Check sheet for the modelled part. Datum: model origin and axes. Units: mm. A direction names the side the tool comes from. Round coordinates to 2 decimals unless told otherwise and drop trailing zeros. Write each loop counter-clockwise with the first axis right and the second up, starting at its lowest first coordinate (ties: lowest second). Pieces come first, ordered by that corner, then holes. Notation, with made-up numbers: (9, 59.25) -> (38, 59.25) arc R26 cw to (38, 90.25) -> close; hole circle Ø10 at (-19, 36.25). An arc over 180 degrees is marked (long way). Write item = value, one per line.
from build123d import *

# Parameters (mm, degrees)
SKETCH1_W                    = 35
SKETCH1_H                    = 35
SKETCH1_R                    = 2.25
BASE_FLANGE1_DEPTH           = 3
EDGE_FLANGE1_DEPTH           = 35
SKETCH9_W                    = 36
SKETCH9_H                    = 35
BOSS_EXTRUDE1_DEPTH          = 3
EDGE_FLANGE2_STRIP_W         = 18
EDGE_FLANGE2_STRIP_H         = 3
EDGE_FLANGE2_STRIP_CUT_DEPTH = 75
EDGE_FLANGE2_DEPTH           = 75
EDGE_FLANGE3_STRIP_W         = 18
EDGE_FLANGE3_STRIP_H         = 3
EDGE_FLANGE3_STRIP_CUT_DEPTH = 75
EDGE_FLANGE3_DEPTH           = 75
SKETCH16_R                   = 5.25
SKETCH16_R_2                 = 1.75
CUT_EXTRUDE1_DEPTH           = 10
BODY_MOVE_COPY1_ANGLE        = 180


# Sheet-metal steps are written as plain solids
with BuildPart() as part:
    # Sketch1 → Base-Flange1 (new body)
    with BuildSketch(Plane.XY):
        Rectangle(SKETCH1_W, SKETCH1_H)
        with Locations((-13, 13)):
            Circle(SKETCH1_R, mode=Mode.SUBTRACT)
        with Locations((13, 13)):
            Circle(SKETCH1_R, mode=Mode.SUBTRACT)
        with Locations((13, -13)):
            Circle(SKETCH1_R, mode=Mode.SUBTRACT)
        with Locations((-13, -13)):
            Circle(SKETCH1_R, mode=Mode.SUBTRACT)
    extrude(amount=-BASE_FLANGE1_DEPTH)

    # Edge-Flange1 section (across the edge) → Edge-Flange1 (add)
    with BuildSketch(Plane(origin=(-17.5, -20.5, 0), x_dir=(0, 1, 0), z_dir=(1, 0, 0))):
        with BuildLine():
            Line((-3, 3), (-3, 17))
            Line((-3, 17), (0, 17))
            Line((0, 17), (0, 3))
            ThreePointArc((0, 3), (0.878679656, 0.878679656), (3, 0))
            Line((3, 0), (3, -3))
            ThreePointArc((3, -3), (-1.242640687, -1.242640687), (-3, 3))
        make_face()
    extrude(amount=EDGE_FLANGE1_DEPTH)

    # Sketch9 → Boss-Extrude1 (add)
    with BuildSketch(Plane.XZ.offset(23.5)):
        Polygon((57.5, 17), (17.5, 17), (17.5, 7), (21.5, 7), (57.5, 7), align=None)
        with Locations((39.5, -10.5)):
            Rectangle(SKETCH9_W, SKETCH9_H)
    extrude(amount=-BOSS_EXTRUDE1_DEPTH)

    # Edge-Flange2 strip (across the edge) → Edge-Flange2 strip cut (cut)
    with BuildSketch(Plane(origin=(57.5, -23.5, 17), x_dir=(0, 0, -1), z_dir=(-1, 0, 0))):
        with Locations((-6, -1.5)):
            Rectangle(EDGE_FLANGE2_STRIP_W, EDGE_FLANGE2_STRIP_H)
    extrude(amount=EDGE_FLANGE2_STRIP_CUT_DEPTH, mode=Mode.SUBTRACT)

    # Edge-Flange2 section (across the edge) → Edge-Flange2 (add)
    with BuildSketch(Plane(origin=(57.5, -23.5, 17), x_dir=(0, 0, -1), z_dir=(-1, 0, 0))):
        with BuildLine():
            Line((-3, 3), (-3, 30))
            Line((-3, 30), (0, 30))
            Line((0, 30), (0, 3))
            ThreePointArc((0, 3), (0.878679656, 0.878679656), (3, 0))
            Line((3, 0), (3, -3))
            ThreePointArc((3, -3), (-1.242640687, -1.242640687), (-3, 3))
        make_face()
    extrude(amount=EDGE_FLANGE2_DEPTH)

    # Edge-Flange3 strip (across the edge) → Edge-Flange3 strip cut (cut)
    with BuildSketch(Plane(origin=(-17.5, -53.5, 20), x_dir=(0, 1, 0), z_dir=(1, 0, 0))):
        with Locations((-6, -1.5)):
            Rectangle(EDGE_FLANGE3_STRIP_W, EDGE_FLANGE3_STRIP_H)
    extrude(amount=EDGE_FLANGE3_STRIP_CUT_DEPTH, mode=Mode.SUBTRACT)

    # Edge-Flange3 section (across the edge) → Edge-Flange3 (add)
    with BuildSketch(Plane(origin=(-17.5, -53.5, 20), x_dir=(0, 1, 0), z_dir=(1, 0, 0))):
        with BuildLine():
            Line((-3, 3), (-3, 46))
            Line((-3, 46), (0, 46))
            Line((0, 46), (0, 3))
            ThreePointArc((0, 3), (0.878679656, 0.878679656), (3, 0))
            Line((3, 0), (3, -3))
            ThreePointArc((3, -3), (-1.242640687, -1.242640687), (-3, 3))
        make_face()
    extrude(amount=EDGE_FLANGE3_DEPTH)

    # Sketch16 → Cut-Extrude1 (cut)
    with BuildSketch(Plane(origin=(0, -20.5, 0), x_dir=(1, 0, 0), z_dir=(0, 1, 0))):
        with Locations(Location((40.5, 17.3, 0), (0, 0, 270))):
            Circle(SKETCH16_R)
        with Locations(Location((40.5, 9.3, 0), (0, 0, 270))):
            Circle(SKETCH16_R_2)
        with Locations(Location((48.5, 17.3, 0), (0, 0, 270))):
            Circle(SKETCH16_R_2)
        with Locations(Location((32.5, 17.3, 0), (0, 0, 270))):
            Circle(SKETCH16_R_2)
    extrude(amount=-CUT_EXTRUDE1_DEPTH, mode=Mode.SUBTRACT)


with BuildPart() as part_1:
    # Body-Move/Copy1: moved
    add(part.part.moved(Location((0, 0, 0))).rotate(Axis((20, -19.25, 19.25), (-4.937700262163626e-15, 0.7071067811864181, 0.707106781186677)), BODY_MOVE_COPY1_ANGLE))


solid = part_1.part
(1) Sectioned sample at C-C on y = -55.8. Enter the section's corners in (x, z), then the cut area to 3 significant figures.
Worked answers:
outline = (-17.5, 15) -> (-10.25, 15) -> (-10.25, 18) -> (-17.5, 18) -> close; (-6.75, 15) -> (-5.75, 15) -> (-5.75, 18) -> (-6.75, 18) -> close; (4.75, 15) -> (5.75, 15) -> (5.75, 18) -> (4.75, 18) -> close; (9.25, 15) -> (18.5, 15) -> (18.5, 18) -> (9.25, 18) -> close
area = 55.5 mm²
(2) Access from +Z, -Z, +X, -X, +Y, -Y to the whole of each face (thin tool, end or side, straight path). Record for faces 5 (the flat face through (19, -21.5, 0)), 6 (the flat face through (19, -18.5, 0)), 7 (the flat face through (21, -31.5, 16)).
Worked answers:
face_5 = -Z, +X, -X, -Y
face_6 = +Z, +X, -X, +Y
face_7 = +Z, -Z, -Y
(3) Material ranges on L1, parallel to X at y = -55.8, z = 17.05; L2, parallel to X at y = -39.1, z = 25.5; L3, parallel to Y at x = 0, z = 17, recorded low to high. Write a range as [from, to].
Worked answers:
L1 = [-17.5, -10.25], [-6.75, -5.75], [4.75, 5.75], [9.25, 18.5]
L2 = [22.5, 24.75], [29.25, 50.75], [55.25, 57.5]
L3 = [-66.5, -61.03], [-50.57, -49.48], [-46.12, -21.18]
(4) Release check for a two-part mould opening along Y. For faces 1 (the cylindrical face through (-0.731, -61.045, 16.521)), 2 (the cylindrical face through (20.525, -19.789, -16.196)), 3 (the flat face through (40, -38.5, 39)), 4 (the cylindrical face through (-7.83, -54.183, 16.521)) record: pulls with the +Y half, pulls with the -Y half, needs draft (parallel to the pull), parting line crosses it, or undercut.
Worked answers:
face_1 = undercut
face_2 = pulls with the -Y half
face_3 = pulls with the +Y half
face_4 = undercut
(5) Sectioned sample at D-D on x = 7.5. Enter the section's corners in (y, z), then the cut area to 3 significant figures.
Worked answers:
outline = (-66.5, 15) -> (-57.55, 15) -> (-57.55, 18) -> (-66.5, 18) -> close; (-54.05, 15) -> (-24.5, 15) arc R3 cw to (-21.5, 12) -> (-21.5, -12) arc R6 ccw to (-15.5, -18) -> (27.5, -18) -> (27.5, -15) -> (-15.5, -15) arc R3 cw to (-18.5, -12) -> (-18.5, 12) arc R6 ccw to (-24.5, 18) -> (-54.05, 18) -> close
area = 359 mm²
(6) Sectioned sample at A-A on x = 27. Enter the section's corners in (y, z).
Worked answers:
outline = (-41.5, 21) arc R6 ccw to (-35.5, 15) -> (-24.5, 15) arc R3 cw to (-21.5, 12) -> (-21.5, -12) arc R6 ccw to (-15.5, -18) -> (27.5, -18) -> (27.5, -15) -> (-15.5, -15) arc R3 cw to (-18.5, -12) -> (-18.5, 12) arc R6 ccw to (-24.5, 18) -> (-35.5, 18) arc R3 cw to (-38.5, 21) -> (-38.5, 23.25) -> (-41.5, 23.25) -> close; (-41.5, 27.75) -> (-38.5, 27.75) -> (-38.5, 49.25) -> (-41.5, 49.25) -> close; (-41.5, 53.75) -> (-38.5, 53.75) -> (-38.5, 56) -> (-41.5, 56) -> close
(7) Go/stop test with flat-tipped pins: P1, Ø1.5, axis at y = -42, z = 16.5, coming from the +X side; P2, Ø12, axis at x = 1.5, z = 5, coming from the +Y side; P3, Ø12.5, axis at x = 35.5, y = -39, coming from the -Z side; P4, Ø4, axis at y = -44.5, z = 12, coming from the +X side. Record where each tip stops, or that it passes through.
Worked answers:
P1 = 18.5
P2 = -18.5
P3 = 15
P4 = through
(8) Sectioned sample at B-B on z = 25.5. Enter the section's corners in (x, y).
Worked answers:
outline = (22.5, -41.5) -> (24.75, -41.5) -> (24.75, -38.5) -> (22.5, -38.5) -> close; (29.25, -41.5) -> (50.75, -41.5) -> (50.75, -38.5) -> (29.25, -38.5) -> close; (55.25, -41.5) -> (57.5, -41.5) -> (57.5, -38.5) -> (55.25, -38.5) -> close
